The drawing under review shows one solid part. Ordinate dimensions are in mm from its lowest x, y, z. A direction names the side the tool comes from. Round coordinates to 2 decimals unless told otherwise and drop trailing zeros. Write each loop counter-clockwise with the first axis right and the second up, starting at its lowest first coordinate (ties: lowest second). Pieces come first, ordered by that corner, then holes. Notation, with made-up numbers: (67.5, 37) -> (103.5, 37) arc R18 ccw to (103.5, 61) -> close; hole circle Ø3 at (-24, 86.25). An arc over 180 degrees is marked (long way). Answer in a Markdown table with one row per item.
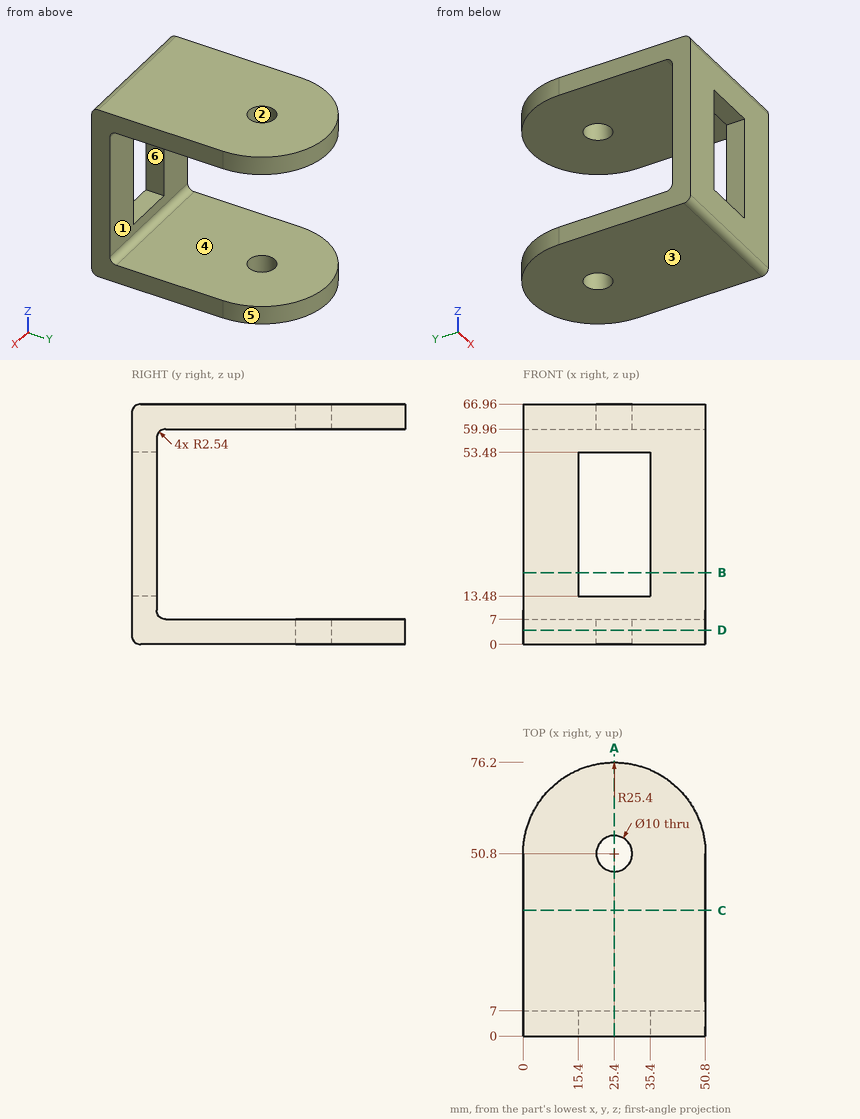
1) For line 1 (Z direction, x = 12, y = 72); line 2 (Z direction, x = 33.5, y = 4); line 3 (Y direction, x = 25, z = 4), list the stretches that pass through material, from the lowest coordinate up. Write a range as [from, to].
Solved:
| item | result |
|---|---|
| line 1 | [0, 7], [59.96, 66.96] |
| line 2 | [0, 13.48], [53.48, 66.96] |
| line 3 | [0, 45.82], [55.78, 76.2] |
2) For the marked faces 4, 5 and 6, list the 3-axis set-ups (+Z, -Z, +X, -X, +Y, -Y) from which the entire face can be reached by the end or side of a thin tool; tool diameter is ignored.
Solved:
| item | result |
|---|---|
| face 4 | +X, -X, +Y |
| face 5 | +Z, -Z, +Y |
| face 6 | +Y, -Y |
3) Mouldability with a two-part tool opening along Z and no side actions: class the marked faces 1, 2 and 3 as pulls with the +Z half, pulls with the -Z half, needs draft (parallel to the pull), parting line crosses it, or undercut.
Solved:
| item | result |
|---|---|
| face 1 | undercut |
| face 2 | needs draft |
| face 3 | pulls with the -Z half |
4) Consider section D-D on z = 4. State the section outline as (x, y) points, then the cut area to 3 significant figures.
Solved:
| item | result |
|---|---|
| outline | (0, 0) -> (50.8, 0) -> (50.8, 50.8) arc R25.4 ccw to (0, 50.8) -> close; hole circle Ø10 at (25.4, 50.8) |
| area | 3,520 mm² |
5) Consider section C-C on y = 35. State the section outline as (x, z) points.
Solved:
| item | result |
|---|---|
| outline | (0, 0) -> (50.8, 0) -> (50.8, 7) -> (0, 7) -> close; (0, 59.96) -> (50.8, 59.96) -> (50.8, 66.96) -> (0, 66.96) -> close |
6) Clearance check with flat-ended pins moving along their axes: pin 1 Ø5.5 at (x, y) = (23.5, 2) entering from -Z; pin 2 Ø5 at (x, z) = (36.5, 45) entering from +Y; pin 3 Ø6 at (y, z) = (18.5, 10.5) entering from -X (3 decimals). State where each tip first meets the part, or that it passes through.
Solved:
| item | result |
|---|---|
| pin 1 | z = 0 |
| pin 2 | y = 7 |
| pin 3 | through |
7) Consider section A-A on x = 25.4. State the section outline as (y, z) points, then the cut area to 3 significant figures.
Solved:
| item | result |
|---|---|
| outline | (0, 2.54) arc R2.54 ccw to (2.54, 0) -> (45.8, 0) -> (45.8, 7) -> (9.54, 7) arc R2.54 cw to (7, 9.54) -> (7, 13.48) -> (0, 13.48) -> close; (0, 53.48) -> (7, 53.48) -> (7, 57.42) arc R2.54 cw to (9.54, 59.96) -> (45.8, 59.96) -> (45.8, 66.96) -> (2.54, 66.96) arc R2.54 ccw to (0, 64.42) -> close; (55.8, 0) -> (76.2, 0) -> (76.2, 7) -> (55.8, 7) -> close; (55.8, 59.96) -> (76.2, 59.96) -> (76.2, 66.96) -> (55.8, 66.96) -> close |
| area | 1,020 mm² |
8) Consider section B-B on z = 20. State the section outline as (x, y) points, then the cut area to 3 significant figures.
Solved:
| item | result |
|---|---|
| outline | (0, 0) -> (15.4, 0) -> (15.4, 7) -> (0, 7) -> close; (35.4, 0) -> (50.8, 0) -> (50.8, 7) -> (35.4, 7) -> close |
| area | 216 mm² |
